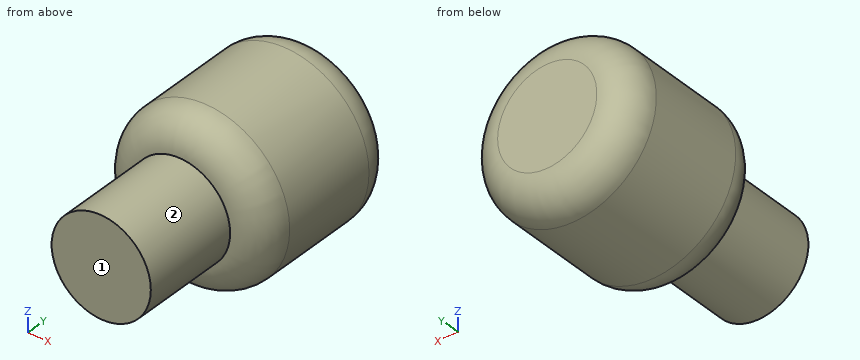
from build123d import *

# Parameters (mm, degrees)
F0_R      = 12.7
F1_DEPTH  = 25.4
F2_R      = 5.08
F3_R      = 6.35
F1_FACE_R = 7.62
F4_DEPTH  = 15.24


with BuildPart() as f1:
    # F0 (on Front) → F1 (new body)
    with BuildSketch(Plane.XZ):
        Circle(F0_R)
    extrude(amount=F1_DEPTH)

    # F2
    f2_edges = [f1.edges().sort_by_distance(p)[0] for p in [
        (-12.7, -25.4, 0),
        (-12.7, 0, 0),
    ]]
    fillet(f2_edges, radius=F2_R)

    # F3 (on Front) + F1_face (on face) → F4 (join)
    with BuildSketch(Plane.XZ):
        Circle(F3_R)
    with BuildSketch(Plane.XZ.offset(25.4)):
        Circle(F1_FACE_R)
    extrude(amount=F4_DEPTH)


solid = f1.part
Can you work these out from the model? Positions are in its coordinate system, mm. Face numbers are marked on the shaded views. A direction names the side the tool comes from. Give positions to 0.01 mm unless a question says otherwise; leave off trailing zeros. Loops run counter-clockwise (first coordinate to the right, second up) from the corner with the lowest first, then second, coordinate; pieces in that order, holes last. Notation, with made-up numbers: M -34,-38.75 L 2,-38.75 A31 ccw 2,-7.75 Z; hole C 78,-6 d9. An arc over 180 degrees is marked long. One line per item, written item: value.
1) I'm going to push flat-ended pins straight in: pin 1 (3 mm diameter, centred on x = -8, y = -33.5, fed in from +Z); pin 2 (3 mm diameter, centred on x = -10, y = -8.5, fed in from +Z); pin 3 (8 mm diameter, centred on x = -2.5, y = -36, fed in from -Z). Where does each tip first touch, or does it pass through?
Geometry check:
pin 1: stops at z = 3.98
pin 2: stops at z = 9.44
pin 3: stops at z = -7.62
2) Imagine slicing it at C-C on y = -28. Write out the boundary of the cut face in (x, z), and give its area (3 significant figures).
Geometry check:
outline: C 0,0 d15.24
area: 182 mm²
3) Imagine slicing it at D-D on y = -12. Write out the boundary of the cut face in (x, z), and give its area (3 significant figures).
Geometry check:
outline: C 0,0 d25.4
area: 507 mm²
4) Please list where these lines run through material, in increasing order: line 1 (Y direction, x = 2.5, z = 7.5); line 2 (X direction, y = -3, z = -10.25); line 3 (Z direction, x = -4.5, y = -36.5).
Geometry check:
line 1: y = -25.39 to -0.01
line 2: x = -6.72 to 6.72
line 3: z = -6.15 to 6.15
5) Imagine slicing it at B-B on z = 0. Write out the boundary of the cut face in (x, y), and give its area (3 significant figures).
Geometry check:
outline: M -12.7,-20.32 A5.08 ccw -7.62,-25.4 L -7.62,-40.64 L 7.62,-40.64 L 7.62,-25.4 A5.08 ccw 12.7,-20.32 L 12.7,-5.08 A5.08 ccw 7.62,0 L -7.62,0 A5.08 ccw -12.7,-5.08 Z
area: 855 mm²
6) On a 3-axis mill with a long thin cutter (end or side, diameter ignored), from which of +Z, -Z, +X, -X, +Y, -Y can I reach the whole of each face in a straight line? I mean the marked faces 1 and 2. Say none if no direction works.
Geometry check:
face 1: +Z, -Z, +X, -X, -Y
face 2: -Y
7) Imagine slicing it at A-A on x = 0. Write out the boundary of the cut face in (y, z), and give its area (3 significant figures).
Geometry check:
outline: M -40.64,-7.62 L -25.4,-7.62 A5.08 ccw -20.32,-12.7 L -5.08,-12.7 A5.08 ccw 0,-7.62 L 0,7.62 A5.08 ccw -5.08,12.7 L -20.32,12.7 A5.08 ccw -25.4,7.62 L -40.64,7.62 Z
area: 855 mm²
